```python
from build123d import *

# Parameters (mm, degrees)
SKETCH2_R           = 2.5
SKETCH2_R_2         = 2
BOSS_EXTRUDE1_DEPTH = 10
SKETCH3_R           = 9.75
BOSS_EXTRUDE2_DEPTH = 30
CUT_EXTRUDE1_REACH  = 32
SKETCH4_R           = 8.5


with BuildPart() as part:
    # Sketch2 → Boss-Extrude1 (new body)
    with BuildSketch(Plane(origin=(0, 0, 0), x_dir=(1, 0, 0), z_dir=(0, 1, 0))):
        with BuildLine():
            Line((0, 7.5), (100, 7.5))
            ThreePointArc((100, 7.5), (107.5, 0), (100, -7.5))
            Line((100, -7.5), (0, -7.5))
            ThreePointArc((0, -7.5), (-7.5, 0), (0, 7.5))
        make_face()
        Circle(SKETCH2_R, mode=Mode.SUBTRACT)
        with Locations((100, 0)):
            Circle(SKETCH2_R_2, mode=Mode.SUBTRACT)
    extrude(amount=BOSS_EXTRUDE1_DEPTH)

    # Sketch3 → Boss-Extrude2 (add)
    with BuildSketch(Plane(origin=(0, 10, 0), x_dir=(-1, 0, 0), z_dir=(0, -1, 0))):
        Circle(SKETCH3_R)
    extrude(amount=BOSS_EXTRUDE2_DEPTH)

    # Sketch4 → Cut-Extrude1 (cut, up to next)
    with BuildSketch(Plane(origin=(0, 10, 0), x_dir=(1, 0, 0), z_dir=(0, 1, 0)), mode=Mode.PRIVATE) as cut_extrude1_sk1:
        Circle(SKETCH4_R)
    cut_extrude1_tool1 = extrude(cut_extrude1_sk1.sketch, amount=-CUT_EXTRUDE1_REACH, mode=Mode.PRIVATE) & part.part
    add(cut_extrude1_tool1.solids().sort_by_distance((0, 10, 0))[0], mode=Mode.SUBTRACT)


solid = part.part
```
Build history of the part. All positions in model axes, mm. A direction names the side the tool comes from. Round coordinates to 2 decimals unless told otherwise and drop trailing zeros. Write each loop counter-clockwise with the first axis right and the second up, starting at its lowest first coordinate (ties: lowest second). Pieces come first, ordered by that corner, then holes.
1) Band-saw the part on A-A, the plane z = 0. List the corners of the cut face in (x, y), and give its area (3 significant figures).
2) Mould opens along Z. For faces 1 (the cylindrical face through (-9.3, -4.79, -2.93)), 2 (the flat face through (54, 5, 7.5)), 3 (the cylindrical face through (101.908, 4.93, -0.601)) say: +Z half, -Z half, draft (parallel to the pull), parting line (faces both ways), or undercut.
3) Drill centre lines: probe 1 along X at (y, z) = (3.25, 0); probe 2 along Z at (x, y) = (0, -12.75); probe 3 along Z at (x, y) = (100, 8). Where is each one in solid material? Low to high.
4) Pin check, flat tips, straight feed: pin 1 (8 mm diameter, centred on x = 52.5, y = -4.5, fed in from -Z); pin 2 (2 mm diameter, centred on x = 50, z = -1.5, fed in from -Y); pin 3 (4 mm diameter, centred on y = -12, z = 2, fed in from +X); pin 4 (5 mm diameter, centred on x = 53, y = 4.5, fed in from -Z). Stop position of each tip, or through.
5) Band-saw the part on D-D, the plane y = 1. List the corners of the cut face in (x, z), and give its area (3 significant figures).
6) Band-saw the part on C-C, the plane y = -6.25. List the corners of the cut face in (x, z).
7) Band-saw the part on B-B, the plane x = 0. List the corners of the cut face in (y, z), and give its area (3 significant figures).
8) 3-axis set-ups, long thin cutter, end or side, ignore diameter. For faces 4 (the flat face through (-1, -20, -9)), 5 (the flat face through (52, 5, -7.5)): which of +Z, -Z, +X, -X, +Y, -Y reach the whole face in a straight line?
Ans:
1. outline: (-9.75, -20) - (-8.5, -20) - (-8.5, 10) - (-9.75, 10) - close; (8.5, -20) - (9.75, -20) - (9.75, 0) - (98, 0) - (98, 10) - (8.5, 10) - close; (102, 0) - (107.5, 0) - (107.5, 10) - (102, 10) - close
1. area: 1,010 mm2
2. face 1: parting line
2. face 2: +Z half
2. face 3: undercut
3. probe 1: x = -9.75 to -8.5, 8.5 to 98, 102 to 107.5
3. probe 2: z = -9.75 to -8.5, 8.5 to 9.75
3. probe 3: z = -7.5 to -2, 2 to 7.5
4. pin 1: passes through
4. pin 2: stops at y = 0
4. pin 3: stops at x = 9.75
4. pin 4: stops at z = -7.5
5. outline: (6.23, -7.5) - (100, -7.5) arc R7.5 ccw to (100, 7.5) - (6.23, 7.5) arc R9.75 ccw (long way) to start; hole circle Ø17 at (0, 0); hole circle Ø4 at (100, 0)
5. area: 1,520 mm2
6. outline: circle Ø19.5 at (0, 0); hole circle Ø17 at (0, 0)
7. outline: (-20, -9.75) - (10, -9.75) - (10, -8.5) - (-20, -8.5) - close; (-20, 8.5) - (10, 8.5) - (10, 9.75) - (-20, 9.75) - close
7. area: 75.0 mm2
8. face 4: +Z, -Z, +X, -X, -Y
8. face 5: -Z, +X, +Y, -Y
